Source: CAD feature listing. Evaluate the final solid. Frame: model axes, mm. A direction names the side the tool comes from. Round coordinates to 2 decimals unless told otherwise and drop trailing zeros. Loops run counter-clockwise (first coordinate to the right, second up) from the corner with the lowest first, then second, coordinate; pieces in that order, holes last. Notation, with made-up numbers: (43.5, 17.25) -> (86.5, 17.25) arc R20 ccw to (86.5, 22.25) -> close; hole circle Ø5 at (-35.5, 14.25). An arc over 180 degrees is marked (long way). Write item = value, one per line.
from build123d import *

# Parameters (mm, degrees)
SKETCH1_W           = 50
SKETCH1_H           = 70.5
SKETCH1_R           = 2.25
SKETCH1_R_2         = 1.6
SKETCH1_R_3         = 4.15
SKETCH1_W_2         = 12
SKETCH1_H_2         = 11
BOSS_EXTRUDE1_DEPTH = 2.5
SKETCH2_W           = 2
SKETCH2_H           = 12
BOSS_EXTRUDE2_DEPTH = 20


with BuildPart() as part:
    # Sketch1 → Boss-Extrude1 (new body)
    with BuildSketch(Plane.XY):
        Rectangle(SKETCH1_W, SKETCH1_H)
        with Locations((-17, 25.25)):
            Circle(SKETCH1_R, mode=Mode.SUBTRACT)
        with Locations((17, 25.25)):
            Circle(SKETCH1_R, mode=Mode.SUBTRACT)
        with Locations((-13.5, -0.25)):
            Circle(SKETCH1_R_2, mode=Mode.SUBTRACT)
        with Locations((13.5, -0.25)):
            Circle(SKETCH1_R_2, mode=Mode.SUBTRACT)
        with Locations((0, -20.25)):
            Circle(SKETCH1_R_3, mode=Mode.SUBTRACT)
        with Locations((0, -0.25)):
            Rectangle(SKETCH1_W_2, SKETCH1_H_2, mode=Mode.SUBTRACT)
    extrude(amount=BOSS_EXTRUDE1_DEPTH)

    # Sketch2 → Boss-Extrude2 (add)
    with BuildSketch(Plane(origin=(0, 0, 0), x_dir=(-1, 0, 0), z_dir=(0, 0, -1))):
        with Locations((6, -20.25)):
            Rectangle(SKETCH2_W, SKETCH2_H)
        with Locations((-6, -20.25)):
            Rectangle(SKETCH2_W, SKETCH2_H)
    extrude(amount=BOSS_EXTRUDE2_DEPTH)


solid = part.part
1. Line query: probe 1 along Y at (x, z) = (17, 0.85); probe 2 along Z at (x, y) = (-21.5, 4.5); probe 3 along X at (y, z) = (-26, -18.25). Output: solid intervals per line, ascending. Write a range as from..to.
Evaluation:
probe_1 = -35.25..23, 27.5..35.25
probe_2 = 0..2.5
probe_3 = -7..-5, 5..7
2. Section query D-D (y = 25.25). Return the cut outline in (x, z).
Evaluation:
outline = (-25, 0) -> (-19.25, 0) -> (-19.25, 2.5) -> (-25, 2.5) -> close; (-14.75, 0) -> (14.75, 0) -> (14.75, 2.5) -> (-14.75, 2.5) -> close; (19.25, 0) -> (25, 0) -> (25, 2.5) -> (19.25, 2.5) -> close
3. Mould query, pull axis Y, two halves, no side actions, for faces 1 (the face through (-6, -14.25, -10)), 2 (the face through (0, 5.25, 1)), 3 (the face through (6, -26.25, -10)), 4 (the face through (7, -20, -10)). Classes: released by +Y, released by -Y, zero draft, split by the parting line, or undercut.
Evaluation:
face_1 = released by +Y
face_2 = undercut
face_3 = released by -Y
face_4 = zero draft
4. Section query C-C (x = -17). Return the cut outline in (y, z), then the cut area to 3 significant figures.
Evaluation:
outline = (-35.25, 0) -> (23, 0) -> (23, 2.5) -> (-35.25, 2.5) -> close; (27.5, 0) -> (35.25, 0) -> (35.25, 2.5) -> (27.5, 2.5) -> close
area = 165 mm²
5. Contact query for flat-ended pins moving along their axis: pin 1 Ø3 at (x, y) = (13.5, -0.25) entering from -Z; pin 2 Ø12 at (x, y) = (15, 8) entering from -Z; pin 3 Ø0.6 at (x, z) = (-6, -10) entering from +Y; pin 4 Ø1 at (x, z) = (-6, -5.5) entering from -Y. Output: stop coordinate, or through.
Evaluation:
pin_1 = through
pin_2 = 0
pin_3 = -14.25
pin_4 = -26.25
6. Section query A-A (z = -10.75). Return the cut outline in (x, y), then the cut area to 3 significant figures.
Evaluation:
outline = (-7, -26.25) -> (-5, -26.25) -> (-5, -14.25) -> (-7, -14.25) -> close; (5, -26.25) -> (7, -26.25) -> (7, -14.25) -> (5, -14.25) -> close
area = 48.0 mm²
7. Set-up query: faces 5 (the face through (5, -20, -10)), 6 (the face through (-6, -26.25, -10)), 7 (the face through (6, -14.25, -10)), 8 (the face through (-7, -20, -10)). Return all of +Z, -Z, +X, -X, +Y, -Y with unobstructed straight access to the full face (end or side cutting, diameter ignored); none if empty.
Evaluation:
face_5 = -Z, +Y, -Y
face_6 = -Z, +X, -X, -Y
face_7 = -Z, +X, -X, +Y
face_8 = -Z, -X, +Y, -Y
8. Section query B-B (y = -0.25). Return the cut outline in (x, z), then the cut area to 3 significant figures.
Evaluation:
outline = (-25, 0) -> (-15.1, 0) -> (-15.1, 2.5) -> (-25, 2.5) -> close; (-11.9, 0) -> (-6, 0) -> (-6, 2.5) -> (-11.9, 2.5) -> close; (6, 0) -> (11.9, 0) -> (11.9, 2.5) -> (6, 2.5) -> close; (15.1, 0) -> (25, 0) -> (25, 2.5) -> (15.1, 2.5) -> close
area = 79.0 mm²
